Part model, mm, in its own coordinate system. A direction names the side the tool comes from. Give positions to 0.01 mm unless a question says otherwise; leave off trailing zeros. Order: outer loops, then holes, each group sorted by start corner. A loop starts at its lowest first (then second) coordinate and runs counter-clockwise, first axis right, second up. Notation, with made-up numbers: (48.5, 44) - (98.5, 44) arc R30 cw to (98.5, 73) - close; hole circle Ø3 at (52.25, -12). An arc over 180 degrees is marked (long way). Use a Markdown table: item, result. Add a question column.
from build123d import *

# Parameters (mm, degrees)
SKETCH_1_W          = 30
SKETCH_1_H          = 117
EXTRUDE_1_DEPTH     = 3
SKETCH_2_R          = 5
CUT_EXTRUDE_1_DEPTH = 1
SKETCH_3_W          = 1.351446616
SKETCH_3_H          = 8.058414564
CUT_EXTRUDE_2_DEPTH = 1
SKETCH_4_W          = 8.25
SKETCH_4_H          = 95.5
SKETCH_4_W_2        = 7
EXTRUDE_2_DEPTH     = 12
EXTRUDE_3_DEPTH     = 2.5


with BuildPart() as part:
    # 草图1 → 凸台-拉伸1 (new body)
    with BuildSketch(Plane.XY):
        Rectangle(SKETCH_1_W, SKETCH_1_H)
    extrude(amount=EXTRUDE_1_DEPTH)

    # 草图2 → 切除-拉伸1 (cut)
    with BuildSketch(Plane.XY.offset(3)):
        with BuildLine():
            Line((-7.5, -35), (-7.5, 35))
            ThreePointArc((-7.5, 35), (0, 42.5), (7.5, 35))
            Line((7.5, 35), (7.5, -35))
            ThreePointArc((7.5, -35), (0, -42.5), (-7.5, -35))
        make_face()
        with Locations((0, -25)):
            Circle(SKETCH_2_R, mode=Mode.SUBTRACT)
    extrude(amount=-CUT_EXTRUDE_1_DEPTH, mode=Mode.SUBTRACT)

    # 草图3 → 切除-拉伸2 (cut)
    with BuildSketch(Plane.XY.offset(3)):
        with Locations((0, -25)):
            Rectangle(SKETCH_3_W, SKETCH_3_H)
    extrude(amount=-CUT_EXTRUDE_2_DEPTH, mode=Mode.SUBTRACT)

    # 草图4 → 凸台-拉伸2 (add)
    with BuildSketch(Plane(origin=(0, 0, 0), x_dir=(-1, 0, 0), z_dir=(0, 0, -1))):
        with Locations((-7.625, 0)):
            Rectangle(SKETCH_4_W, SKETCH_4_H)
        Rectangle(SKETCH_4_W_2, SKETCH_4_H)
        with BuildLine():
            Line((-3.5, 52.25), (-3.5, 47.75))
            Line((-3.5, 47.75), (3.5, 47.75))
            Line((3.5, 47.75), (3.5, 52.25))
            ThreePointArc((3.5, 52.25), (0, 55.75), (-3.5, 52.25))
        make_face()
        with Locations((7.625, 0)):
            Rectangle(SKETCH_4_W, SKETCH_4_H)
        with BuildLine():
            Line((3.5, -47.75), (-3.5, -47.75))
            Line((-3.5, -47.75), (-3.5, -52.25))
            ThreePointArc((-3.5, -52.25), (0, -55.75), (3.5, -52.25))
            Line((3.5, -52.25), (3.5, -47.75))
        make_face()
    extrude(amount=EXTRUDE_2_DEPTH)

    # 草图5 → 凸台-拉伸3 (add)
    with BuildSketch(Plane(origin=(0, 0, -12), x_dir=(-1, 0, 0), z_dir=(0, 0, -1))):
        with BuildLine():
            Line((0, 52.25), (51, 52.25))
            ThreePointArc((51, 52.25), (54.535533906, 50.785533906), (56, 47.25))
            Line((56, 47.25), (56, 42.25))
            ThreePointArc((56, 42.25), (54.535533906, 38.714466094), (51, 37.25))
            Line((51, 37.25), (0, 37.25))
            Line((0, 37.25), (0, 52.25))
        make_face()
    extrude(amount=EXTRUDE_3_DEPTH)


solid = part.part
1. Mould opens along Z. For faces 1 (the face through (3.5, 50, -6)), 2 (the face through (-28, 45, -14.5)), 3 (the face through (-3.5, 50, -6)) say: released by +Z, released by -Z, zero draft, split by the parting line, or undercut.
2. Cut at B-B (z = -2.75). Write the cut outline in (x, y), plus the area to 3 significant figures.
3. Cut at A-A (y = -25). Write the cut outline in (x, z).
4. Pin check, flat tips, straight feed: P1, Ø4, axis at y = 14, z = -4, coming from the -X side; P2, Ø3, axis at y = 6.5, z = -6, coming from the +X side; P3, Ø8, axis at x = -37, z = -11.5, coming from the +Y side. Stop position of each tip, or through.
5. Cut at C-C (x = -25). Write the cut outline in (y, z).
6. Cut at D-D (y = -50.5). Write the cut outline in (x, z), plus the area to 3 significant figures.
7. Drill centre lines: probe 1 along X at (y, z) = (7.5, -11.25); probe 2 along Y at (x, z) = (-5.5, -9.25); probe 3 along Z at (x, y) = (6, 41.5). Where is each one in solid material? Low to high. Write a range as [from, to].
8. Tool access for faces 4 (the face through (0.16, -42.5, 2.51)), 5 (the face through (-3.5, -50, -6)), 6 (the face through (-15, -1, 1)): list every direction of +Z, -Z, +X, -X, +Y, -Y with a clear straight run to the whole face (end or side of a thin tool).
Responses:
| question | item | result |
|---|---|---|
| 1 | face 1 | zero draft |
| 1 | face 2 | released by -Z |
| 1 | face 3 | undercut |
| 2 | outline | (-11.75, -47.75) - (-3.5, -47.75) - (-3.5, -52.25) arc R3.5 ccw to (3.5, -52.25) - (3.5, -47.75) - (11.75, -47.75) - (11.75, 47.75) - (3.5, 47.75) - (3.5, 52.25) arc R3.5 ccw to (-3.5, 52.25) - (-3.5, 47.75) - (-11.75, 47.75) - close |
| 2 | area | 2,350 mm² |
| 3 | outline | (-15, 0) - (-11.75, 0) - (-11.75, -12) - (11.75, -12) - (11.75, 0) - (15, 0) - (15, 3) - (7.5, 3) - (7.5, 2) - (5, 2) - (5, 3) - (0.68, 3) - (0.68, 2) - (-0.68, 2) - (-0.68, 3) - (-5, 3) - (-5, 2) - (-7.5, 2) - (-7.5, 3) - (-15, 3) - close |
| 4 | P1 | stops at x = -11.75 |
| 4 | P2 | stops at x = 11.75 |
| 4 | P3 | stops at y = 52.25 |
| 5 | outline | (37.25, -14.5) - (52.25, -14.5) - (52.25, -12) - (37.25, -12) - close |
| 6 | outline | (-15, 0) - (-3.5, 0) - (-3.5, -12) - (3.5, -12) - (3.5, 0) - (15, 0) - (15, 3) - (-15, 3) - close |
| 6 | area | 174 mm² |
| 7 | probe 1 | x = [-11.75, 11.75] |
| 7 | probe 2 | y = [-47.75, 47.75] |
| 7 | probe 3 | z = [-12, 3] |
| 8 | face 4 | +Z |
| 8 | face 5 | -Z, -X, -Y |
| 8 | face 6 | +Z, -X, +Y, -Y |
